Autodesk Inventor part; units mm, degrees
ref_plane "YZ Plane" through (0, 0, 0) normal (1, 0, 0) x (0, 1, 0)
ref_plane "XZ Plane" through (0, 0, 0) normal (0, 1, 0) x (-1, 0, 0)
ref_plane "XY Plane" through (0, 0, 0) normal (0, 0, 1) x (1, 0, 0)
sketch "草图1" plane through (0, 0, 0) normal (0, 0, 1) x (1, 0, 0)
  line L0 (32, -20) -> (-32, -20)
  line L1 (-32, -20) -> (-32, 20)
  line L2 (-32, 20) -> (32, 20)
  line L3 (32, 20) -> (32, -20)
  line L4 (32, -20) -> (-32, 20) construction
  line L5 (-32, -20) -> (32, 20) construction
  line L6 (-32, 10) -> (-30, 10)
  line L7 (-30, 10) -> (-30, -20)
  line L8 (-30, -20) -> (-32, -20)
  line L9 (-32, -20) -> (-32, 10)
  point P0 (0, 0)
  dimension "d0" = 64
  dimension "d1" = 40
  dimension "d2" = 2
  dimension "d3" = 30
extrude "拉伸1" add sketch "草图1" along normal blind 3
sketch "草图3" plane through (0, 0, 3) normal (0, 0, 1) x (1, 0, 0)
  circle A0 centre (-27, 5) radius 1
  line L0 (-32, 20) -> (-32, -20)
  line L1 (32, 20) -> (-32, 20)
  circle A1 centre (-2, 7) radius 1
  circle A2 centre (15, 3) radius 1
  circle A3 centre (29, 2) radius 1
  line L2 (32, -20) -> (32, 20)
  point P0 (0, 0)
  dimension "d10" = 2
  dimension "d11" = 5
  dimension "d12" = 15
  dimension "d13" = 2
  dimension "d14" = 25
  dimension "d16" = 2
  dimension "d17" = 2
  dimension "d19" = 4
  dimension "d20" = 17
  dimension "d21" = 2
  dimension "d22" = 1
  dimension "d23" = 3
  dimension "d24" = 14
extrude "拉伸2" cut sketch "草图3" against normal blind 10
sketch "草图4" plane through (0, 0, 3) normal (0, 0, 1) x (1, 0, 0)
  line L0 (-30, 18.1876) -> (-19, 18.1876)
  line L1 (-19, 18.1876) -> (-19, 8.1876)
  line L2 (-19, 8.1876) -> (-30, 8.1876)
  line L3 (-30, 8.1876) -> (-30, 18.1876)
  line L4 (-32, 20) -> (-32, -20)
  point P0 (0, 0)
  dimension "d27" = 2
  dimension "d28" = 10
  dimension "d29" = 11
extrude "拉伸3" add sketch "草图4" along normal blind 1
sketch "草图5" plane through (0, 0, 3) normal (0, 0, 1) x (1, 0, 0)
  point P0 (0, 0)
properties part number "摄像头电路部分"
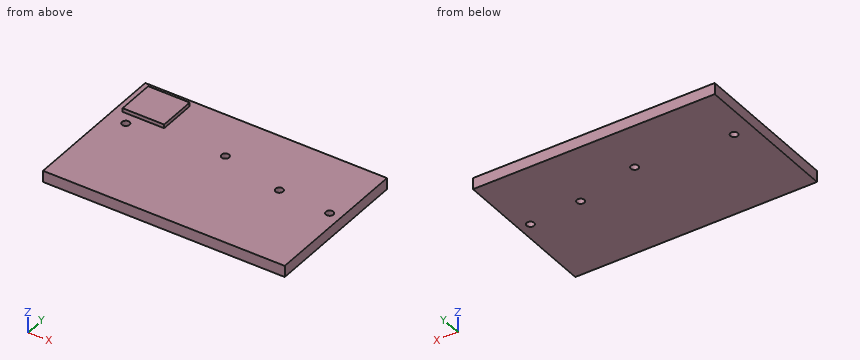
CAD build for the part. Positions are in the model's coordinates, mm. Give positions to 0.01 mm unless a question says otherwise; leave off trailing zeros. Write each loop counter-clockwise with the first axis right and the second up, starting at its lowest first coordinate (ties: lowest second). Pieces come first, ordered by that corner, then holes. Notation, with made-up numbers: (-15.75, -23.75) - (-10.75, -23.75) arc R31 cw to (-10.75, 4.25) - close; hole circle Ø3 at (73, 82.5). An arc over 180 degrees is marked (long way). Put each result on its own line as item: value.
(1) Saw through at C-C (y = 15). List the corners of the cut face in (x, z), then the cut area to 3 significant figures.
Working result:
outline: (-32, 0) - (32, 0) - (32, 3) - (-19, 3) - (-19, 4) - (-30, 4) - (-30, 3) - (-32, 3) - close
area: 203 mm^2
(2) Wall check: L1, parallel to Y at x = 29, z = 1.7; L2, parallel to Y at x = 15, z = 2.35; L3, parallel to Z at x = 24, y = -1. Give the ranges that are in metal, low to high.
Working result:
L1: -20 to 1, 3 to 20
L2: -20 to 2, 4 to 20
L3: 0 to 3
(3) Drop flat-ended pins along their axis: pin 1 Ø2.5 at (x, y) = (-27, 5) entering from +Z; pin 2 Ø0.8 at (y, z) = (12.5, 3.5) entering from +X. Give the stop position or say it passes through.
Working result:
pin 1: z = 3
pin 2: x = -19
(4) Saw through at B-B (x = -27). List the corners of the cut face in (y, z), then the cut area to 3 significant figures.
Working result:
outline: (-20, 0) - (4, 0) - (4, 3) - (-20, 3) - close; (6, 0) - (20, 0) - (20, 3) - (18.19, 3) - (18.19, 4) - (8.19, 4) - (8.19, 3) - (6, 3) - close
area: 124 mm^2
(5) Saw through at D-D (x = 1.5). List the corners of the cut face in (y, z).
Working result:
outline: (-20, 0) - (20, 0) - (20, 3) - (-20, 3) - close
(6) Saw through at A-A (y = 7). List the corners of the cut face in (x, z), then the cut area to 3 significant figures.
Working result:
outline: (-32, 0) - (-3, 0) - (-3, 3) - (-32, 3) - close; (-1, 0) - (32, 0) - (32, 3) - (-1, 3) - close
area: 186 mm^2
